```python
from build123d import *

# Parameters (mm, degrees)
SKETCH1_R           = 2
BOSS_EXTRUDE1_DEPTH = 2
CUT_EXTRUDE1_DEPTH  = 1
SKETCH3_R           = 1.1
BOSS_EXTRUDE2_DEPTH = 4


with BuildPart() as part:
    # Sketch1 → Boss-Extrude1 (new body)
    with BuildSketch(Plane(origin=(0, 0, 0), x_dir=(1, 0, 0), z_dir=(0, 1, 0))):
        with Locations(Location((0, 0, 0), (0, 0, 270))):
            Circle(SKETCH1_R)
    extrude(amount=BOSS_EXTRUDE1_DEPTH)

    # Sketch2 → Cut-Extrude1 (cut)
    with BuildSketch(Plane.XZ):
        Polygon((1.30710226, -0.116595976), (0.754526207, 1.073685774), (-0.552576053, 1.190281751), (-1.30710226, 0.116595976), (-0.754526207, -1.073685774), (0.552576053, -1.190281751), align=None)
    extrude(amount=-CUT_EXTRUDE1_DEPTH, mode=Mode.SUBTRACT)

    # Sketch3 → Boss-Extrude2 (add)
    with BuildSketch(Plane(origin=(0, 2, 0), x_dir=(1, 0, 0), z_dir=(0, 1, 0))):
        with Locations(Location((0, 0, 0), (0, 0, 270))):
            Circle(SKETCH3_R)
    extrude(amount=BOSS_EXTRUDE2_DEPTH)


solid = part.part
```
Work out the finished part from the listing and answer in its coordinate system (mm). A direction names the side the tool comes from. Round coordinates to 2 decimals unless told otherwise and drop trailing zeros. Write each loop counter-clockwise with the first axis right and the second up, starting at its lowest first coordinate (ties: lowest second). Pieces come first, ordered by that corner, then holes. Notation, with made-up numbers: (56, 4) - (105, 4) arc R11 cw to (105, 16) - close; hole circle Ø7 at (22.25, 39). An arc over 180 degrees is marked (long way). Return JSON: item names as keys, results as strings. Group by question number.
Q1. The part is cut by section A-A on z = 0. Write down the section's boundary in (x, y), then the cut area to 3 significant figures.
Q2. The mould has two halves that part along X. Classify faces 1 (the flat face through (0, 1, 0)), 2 (the cylindrical face through (-2, 1, 0)), 3 (the flat face through (-1, 0, 1)): released by +X, released by -X, zero draft, split by the parting line, or undercut.
Q3. For faces 4 (the flat face through (-1.035, 0.493, -0.47)), 5 (the flat face through (0, 6, 0)), 6 (the cylindrical face through (1.09, 3.97, -0.14)), determine the directions among +Z, -Z, +X, -X, +Y, -Y from which every point of the face is accessible in a straight line to the end or side of a thin tool.
Q4. The part is cut by section B-B on x = 0.2. Write down the section's boundary in (y, z).
Q5. Find the intervals of material crossed by L1, parallel to Y at x = 0.9, z = 0.35; L2, parallel to Y at x = -1.15, z = -0.4; L3, parallel to X at y = 0.95, z = -0.2, in increasing order.
Q6. The part is cut by section D-D on y = 4.4. Write down the section's boundary in (x, z), then the cut area to 3 significant figures.
Q7. The part is cut by section C-C on y = 1.65. Write down the section's boundary in (x, z).
Q8. Each of these flat-tipped pins is pushed along its axis until it touches: pin 1 Ø1.2 at (x, z) = (0.5, 0) entering from -Y; pin 2 Ø1.5 at (y, z) = (4.5, -1) entering from -X. Where does it stop, or does it pass through?
Solved:
{
 "1": {"outline": "(-2, 0) - (-1.25, 0) - (-1.25, 1) - (1.25, 1) - (1.25, 0) - (2, 0) - (2, 2) - (1.1, 2) - (1.1, 6) - (-1.1, 6) - (-1.1, 2) - (-2, 2) - close", "area": "14.3 mm²"},
 "2": {"face 1": "undercut", "face 2": "split by the parting line", "face 3": "zero draft"},
 "3": {"face 4": "-Y", "face 5": "+Z, -Z, +X, -X, +Y", "face 6": "+Y"},
 "4": {"outline": "(0, -1.99) - (2, -1.99) - (2, -1.08) - (6, -1.08) - (6, 1.08) - (2, 1.08) - (2, 1.99) - (0, 1.99) - (0, 1.12) - (1, 1.12) - (1, -1.16) - (0, -1.16) - close"},
 "5": {"L1": "1 to 6", "L2": "0 to 2", "L3": "-1.99 to -1.16, 1.25 to 1.99"},
 "6": {"outline": "circle Ø2.2 at (0, 0)", "area": "3.80 mm²"},
 "7": {"outline": "circle Ø4 at (0, 0)"},
 "8": {"pin 1": "y = 1", "pin 2": "x = -1.07"}
}
